```python
from build123d import *

# Parameters (mm, degrees)
SKETCH1_W           = 100
SKETCH1_H           = 30
BOSS_EXTRUDE1_DEPTH = 3
SKETCH2_W           = 3
SKETCH2_H           = 30
BOSS_EXTRUDE2_DEPTH = 20
SKETCH3_R           = 2
CUT_EXTRUDE1_DEPTH  = 104.701494685
SKETCH4_R           = 2
CUT_EXTRUDE2_DEPTH  = 10


with BuildPart() as part:
    # Sketch1 → Boss-Extrude1 (new body)
    with BuildSketch(Plane.XY):
        Rectangle(SKETCH1_W, SKETCH1_H)
    extrude(amount=BOSS_EXTRUDE1_DEPTH)

    # Sketch2 → Boss-Extrude2 (add)
    with BuildSketch(Plane.XY.offset(3)):
        with Locations((-48.5, 0)):
            Rectangle(SKETCH2_W, SKETCH2_H)
    extrude(amount=BOSS_EXTRUDE2_DEPTH)

    # Sketch3 → Cut-Extrude1 (cut, through all)
    with BuildSketch(Plane.ZY.offset(50)):
        with Locations((13, 5)):
            Circle(SKETCH3_R)
        with Locations((13, -10)):
            Circle(SKETCH3_R)
    extrude(amount=-CUT_EXTRUDE1_DEPTH, mode=Mode.SUBTRACT)

    # Sketch4 → Cut-Extrude2 (cut)
    with BuildSketch(Plane(origin=(0, 0, 0), x_dir=(-1, 0, 0), z_dir=(0, 0, -1))):
        with Locations((-40, 0)):
            Circle(SKETCH4_R)
    extrude(amount=-CUT_EXTRUDE2_DEPTH, mode=Mode.SUBTRACT)


solid = part.part
```
Could you check a few things on this model? Use its own coordinates, in mm. A direction names the side the tool comes from. Round coordinates to 2 decimals unless told otherwise and drop trailing zeros. Write each loop counter-clockwise with the first axis right and the second up, starting at its lowest first coordinate (ties: lowest second). Pieces come first, ordered by that corner, then holes. Notation, with made-up numbers: M 89.25,-3.75 L 113.25,-3.75 A37 ccw 113.25,33.25 Z; hole C 40,24.25 d11. An arc over 180 degrees is marked long. Answer in a Markdown table with one row per item. Add a question column.
Q1. If I drill on line 1 (Y direction, x = 40, z = 1.9); line 2 (Z direction, x = -0.5, y = -9); line 3 (X direction, y = 7.25, z = 8.5), over which ranges is the centre line in solid material (lowest first)? Write a range as from..to.
Q2. Imagine slicing it at A-A (z = 13). Please give me the cut outline in (x, y).
Q3. Will these pins go through, and if not, where does the flat tip stop? pin 1 Ø10 at (y, z) = (-9, 4) entering from +X; pin 2 Ø5 at (x, y) = (40, 0) entering from +Z; pin 3 Ø6 at (y, z) = (6, 8.5) entering from +X.
Q4. On a 3-axis mill with a long thin cutter (end or side, diameter ignored), from which of +Z, -Z, +X, -X, +Y, -Y can I reach the whole of each face in a straight line? I mean faces 4 (the cylindrical face through (-49, 5, 11)), 5 (the flat face through (1, 0, 3)). Say none if no direction works.
Q5. If we mould it in two halves opening along Y, with no side actions, what happens to faces 1 (the cylindrical face through (-48.521, -8.648, 11.526)), 2 (the flat face through (-8, 15, 2)), 3 (the flat face through (-50, 0, 11))? For each: +Y half, -Y half, draft (parallel to the pull), parting line (faces both ways), or undercut.
Q6. Imagine slicing it at D-D (y = 12.5). Please give me the cut outline in (x, z).
Q7. Imagine slicing it at B-B (x = 40). Please give me the cut outline in (y, z), then the cut area to 3 significant figures.
Q8. Imagine slicing it at C-C (y = 0). Please give me the cut outline in (x, z), then the cut area to 3 significant figures.
Values:
| question | item | result |
|---|---|---|
| 1 | line 1 | -15..-2, 2..15 |
| 1 | line 2 | 0..3 |
| 1 | line 3 | -50..-47 |
| 2 | outline | M -50,-15 L -47,-15 L -47,-12 L -50,-12 Z; M -50,-8 L -47,-8 L -47,3 L -50,3 Z; M -50,7 L -47,7 L -47,15 L -50,15 Z |
| 3 | pin 1 | x = 50 |
| 3 | pin 2 | z = 3 |
| 3 | pin 3 | x = -47 |
| 4 | face 4 | +X, -X |
| 4 | face 5 | +Z, +X, +Y, -Y |
| 5 | face 1 | undercut |
| 5 | face 2 | +Y half |
| 5 | face 3 | draft |
| 6 | outline | M -50,0 L 50,0 L 50,3 L -47,3 L -47,23 L -50,23 Z |
| 7 | outline | M -15,0 L -2,0 L -2,3 L -15,3 Z; M 2,0 L 15,0 L 15,3 L 2,3 Z |
| 7 | area | 78.0 mm^2 |
| 8 | outline | M -50,0 L 38,0 L 38,3 L -47,3 L -47,23 L -50,23 Z; M 42,0 L 50,0 L 50,3 L 42,3 Z |
| 8 | area | 348 mm^2 |
